```python
from build123d import *

# Parameters (mm, degrees)
BASE_FLANGE1_DEPTH = 2
SKETCH2_R          = 5
CUT_EXTRUDE1_DEPTH = 10
SKETCH4_R          = 4
CUT_EXTRUDE3_DEPTH = 10


# Sheet-metal steps are written as plain solids
with BuildPart() as part:
    # Sketch1 → Base-Flange1 (new body)
    with BuildSketch(Plane.XY):
        with BuildLine():
            Line((16.661890932, 10.015815157), (4.161890932, 10.015815157))
            Line((4.161890932, 10.015815157), (-146.015023604, 9.593165426))
            Line((-146.015023604, 9.593165426), (-158.515023604, 9.593165426))
            ThreePointArc((-158.515023604, 9.593165426), (-160.282790557, 10.325398473), (-161.015023604, 12.093165426))
            Line((-161.015023604, 12.093165426), (-161.015023604, 59.149789753))
            ThreePointArc((-161.015023604, 59.149789753), (-160.680087113, 60.399789753), (-159.765023604, 61.314853262))
            Line((-159.765023604, 61.314853262), (-127.954134471, 79.680878666))
            ThreePointArc((-127.954134471, 79.680878666), (-127.351182084, 79.930629722), (-126.704134471, 80.015815157))
            Line((-126.704134471, 80.015815157), (16.661890932, 80.015815157))
            ThreePointArc((16.661890932, 80.015815157), (18.429657885, 79.28358211), (19.161890932, 77.515815157))
            Line((19.161890932, 77.515815157), (19.161890932, 12.515815157))
            ThreePointArc((19.161890932, 12.515815157), (18.429657885, 10.748048204), (16.661890932, 10.015815157))
        make_face()
    extrude(amount=-BASE_FLANGE1_DEPTH)

    # Sketch2 → Cut-Extrude1 (cut)
    with BuildSketch(Plane(origin=(0, 0, -2), x_dir=(-1, 0, 0), z_dir=(0, 0, -1))):
        with Locations((115.97079497, 35.621477589)):
            Circle(SKETCH2_R)
    extrude(amount=-CUT_EXTRUDE1_DEPTH, mode=Mode.SUBTRACT)

    # Sketch4 → Cut-Extrude3 (cut)
    with BuildSketch(Plane.XY):
        with Locations((1.661890932, 25.015815157)):
            Circle(SKETCH4_R)
    extrude(amount=-CUT_EXTRUDE3_DEPTH, mode=Mode.SUBTRACT)


solid = part.part
```
Part model, mm, in its own coordinate system. Give positions to 0.01 mm unless a question says otherwise; leave off trailing zeros. Order: outer loops, then holes, each group sorted by start corner. A loop starts at its lowest first (then second) coordinate and runs counter-clockwise, first axis right, second up. Notation, with made-up numbers: M 77,12.25 L 128,12.25 A29 cw 128,49.25 Z; hole C 40.25,-32 d4. An arc over 180 degrees is marked long. Use a Markdown table: item, result. Add a question column.
(1) Mould opens along Y. For faces 1 (the face through (-144.08, 70.37, -0.99)), 2 (the face through (-70, 45, -2)), 3 (the face through (-120.74, 37.12, -1.01)) say: +Y half, -Y half, draft (parallel to the pull), parting line (faces both ways), or undercut.
(2) Probe line 1 along Y through (x, z) = (-6, -1.85); line 2 along X through (y, z) = (33.5, -0.55); line 3 along X through (y, z) = (22, -0.25). List the from-to ranges inside material, lowest first. Write a range as [from, to].
(3) Saw through at C-C, the plane x = 0. Give the cut face in (y, z).
(4) Saw through at A-A, the plane x = -118. Give the cut face in (y, z).
(5) Saw through at B-B, the plane z = -1.6. Give the cut face in (x, y).
(6) Drop a flat-ended pin along its axis: P1, Ø1, axis at x = 12, z = -0.5, coming from the -Y side. Give the stop position or say it passes through.
Answer key:
| question | item | result |
|---|---|---|
| 1 | face 1 | +Y half |
| 1 | face 2 | draft |
| 1 | face 3 | undercut |
| 2 | line 1 | [9.99, 80.02] |
| 2 | line 2 | [-161.02, -120.5], [-111.44, 19.16] |
| 2 | line 3 | [-161.02, -0.97], [4.29, 19.16] |
| 3 | outline | M 10,-2 L 21.38,-2 L 21.38,0 L 10,0 Z; M 28.65,-2 L 80.02,-2 L 80.02,0 L 28.65,0 Z |
| 4 | outline | M 9.67,-2 L 31.05,-2 L 31.05,0 L 9.67,0 Z; M 40.19,-2 L 80.02,-2 L 80.02,0 L 40.19,0 Z |
| 5 | outline | M -161.02,12.09 A2.5 ccw -158.52,9.59 L -146.02,9.59 L 4.16,10.02 L 16.66,10.02 A2.5 ccw 19.16,12.52 L 19.16,77.52 A2.5 ccw 16.66,80.02 L -126.7,80.02 A2.5 ccw -127.95,79.68 L -159.77,61.31 A2.5 ccw -161.02,59.15 Z; hole C -115.97,35.62 d10; hole C 1.66,25.02 d8 |
| 6 | P1 | y = 10.02 |
